Here's how the part is built. I have some questions about the finished solid (model axes, mm). A direction names the side the tool comes from. Give positions to 0.01 mm unless a question says otherwise; leave off trailing zeros. Loops run counter-clockwise (first coordinate to the right, second up) from the corner with the lowest first, then second, coordinate; pieces in that order, holes last. Notation, with made-up numbers: (56, 79) - (88, 79) arc R21 cw to (88, 115) - close; hole circle Ø9 at (-31.5, -4). An arc over 180 degrees is marked (long way). Use a Markdown table: item, result.
from build123d import *

# Parameters (mm, degrees)
BOSS_EXTRUDE1_DEPTH = 20
SKETCH3_R           = 1.6
CUT_EXTRUDE1_DEPTH  = 20
SKETCH4_R           = 3
CUT_EXTRUDE2_DEPTH  = 4
FILLET5_R           = 2


with BuildPart() as part:
    # Sketch2 → Boss-Extrude1 (new body)
    with BuildSketch(Plane.XY):
        with BuildLine():
            Line((0, 0), (-2, 0))
            Line((-2, 0), (-2, 12))
            Line((-2, 12), (14.9, 12))
            Line((14.9, 12), (14.9, 0))
            Line((14.9, 0), (12.9, 0))
            ThreePointArc((12.9, 0), (6.45, 6.45), (0, 0))
        make_face()
    extrude(amount=-BOSS_EXTRUDE1_DEPTH)

    # Sketch3 → Cut-Extrude1 (cut)
    with BuildSketch(Plane(origin=(0, 12, 0), x_dir=(1, 0, 0), z_dir=(0, 1, 0))):
        with Locations(Location((6.45, 10, 0), (0, 0, 270))):
            Circle(SKETCH3_R)
    extrude(amount=-CUT_EXTRUDE1_DEPTH, mode=Mode.SUBTRACT)

    # Sketch4 → Cut-Extrude2 (cut)
    with BuildSketch(Plane(origin=(0, 12, 0), x_dir=(1, 0, 0), z_dir=(0, 1, 0))):
        with Locations(Location((6.45, 10, 0), (0, 0, 270))):
            Circle(SKETCH4_R)
    extrude(amount=-CUT_EXTRUDE2_DEPTH, mode=Mode.SUBTRACT)

    # Fillet5
    fillet5_edges = [part.edges().sort_by_distance(p)[0] for p in [
        (-2, 12, -10),
        (14.9, 12, -10),
        (6.45, 12, -20),
        (6.45, 12, -13),
        (6.45, 12, 0),
    ]]
    fillet(fillet5_edges, radius=FILLET5_R)


solid = part.part
(1) We'd pull the mould along Z, two halves only. Please class faces 3 (the face through (6.57, 11.4, -0.57)), 4 (the face through (8.48, 9.01, -12.21)), 5 (the face through (14, 0, -10)): pulls with the +Z half, pulls with the -Z half, needs draft (parallel to the pull), parting line crosses it, or undercut.
A:
| item | result |
|---|---|
| face 3 | pulls with the +Z half |
| face 4 | undercut |
| face 5 | needs draft |
(2) On a 3-axis mill with a long thin cutter (end or side, diameter ignored), from which of +Z, -Z, +X, -X, +Y, -Y can I reach the whole of each face in a straight line? I mean faces 1 (the face through (5, 8, -9)), 2 (the face through (-1.43, 11.4, -10.14)). Say none if no direction works.
A:
| item | result |
|---|---|
| face 1 | +Y |
| face 2 | +Z, -Z, -X, +Y |
(3) Suppose I cut it at B-B on x = 6.45. Write out the boundary of the cut face in (y, z), plus the area to 3 significant figures.
A:
| item | result |
|---|---|
| outline | (6.45, -20) - (10, -20) arc R2 ccw to (12, -18) - (12, -15) arc R2 ccw to (10, -13) - (8, -13) - (8, -11.6) - (6.45, -11.6) - close; (6.45, -8.4) - (8, -8.4) - (8, -7) - (10, -7) arc R2 ccw to (12, -5) - (12, -2) arc R2 ccw to (10, 0) - (6.45, 0) - close |
| area | 78.6 mm2 |
(4) If I drill on line 1 (X direction, y = 6.75, z = -10); line 2 (Y direction, x = 13, z = -16.75); line 3 (Z direction, x = 4.5, y = 8.5), over which ranges is the centre line in solid material (lowest first)?
A:
| item | result |
|---|---|
| line 1 | -2 to 4.85, 8.05 to 14.9 |
| line 2 | 0 to 12 |
| line 3 | -20 to -12.28, -7.72 to 0 |
(5) Suppose I cut it at D-D on y = 2.75. Write out the boundary of the cut face in (x, z), plus the area to 3 significant figures.
A:
| item | result |
|---|---|
| outline | (-2, -20) - (0.62, -20) - (0.62, 0) - (-2, 0) - close; (12.28, -20) - (14.9, -20) - (14.9, 0) - (12.28, 0) - close |
| area | 105 mm2 |
(6) Will these pins go through, and if not, where does the flat tip stop? pin 1 (9.5 mm diameter, centred on x = 6.45, z = -10, fed in from +Y); pin 2 (4 mm diameter, centred on x = 6.45, z = -10, fed in from -Y).
A:
| item | result |
|---|---|
| pin 1 | y = 11.98 |
| pin 2 | y = 6.13 |
(7) Suppose I cut it at C-C on y = 7.25. Write out the boundary of the cut face in (x, z), plus the area to 3 significant figures.
A:
| item | result |
|---|---|
| outline | (-2, -20) - (14.9, -20) - (14.9, 0) - (-2, 0) - close; hole circle Ø3.2 at (6.45, -10) |
| area | 330 mm2 |
(8) Suppose I cut it at A-A on z = -10. Write out the boundary of the cut face in (x, y), plus the area to 3 significant figures.
A:
| item | result |
|---|---|
| outline | (-2, 0) - (0, 0) arc R6.45 cw to (4.85, 6.25) - (4.85, 8) - (3.45, 8) - (3.45, 10) arc R2 ccw to (1.45, 12) - (0, 12) arc R2 ccw to (-2, 10) - close; (8.05, 6.25) arc R6.45 cw to (12.9, 0) - (14.9, 0) - (14.9, 10) arc R2 ccw to (12.9, 12) - (11.45, 12) arc R2 ccw to (9.45, 10) - (9.45, 8) - (8.05, 8) - close |
| area | 105 mm2 |
